Check sheet for the drawn part. Datum: minimum x, y, z corner. Units: mm. A direction names the side the tool comes from. Round coordinates to 2 decimals unless told otherwise and drop trailing zeros. Order: outer loops, then holes, each group sorted by start corner. A loop starts at its lowest first (then second) coordinate and runs counter-clockwise, first axis right, second up. Notation, with made-up numbers: (66.25, -32.5) - (119.25, -32.5) arc R5 cw to (119.25, -27.5) - close; hole circle Ø10 at (61, -33). An arc over 180 degrees is marked (long way). Write each question's results on one line, items separated by ' | '.
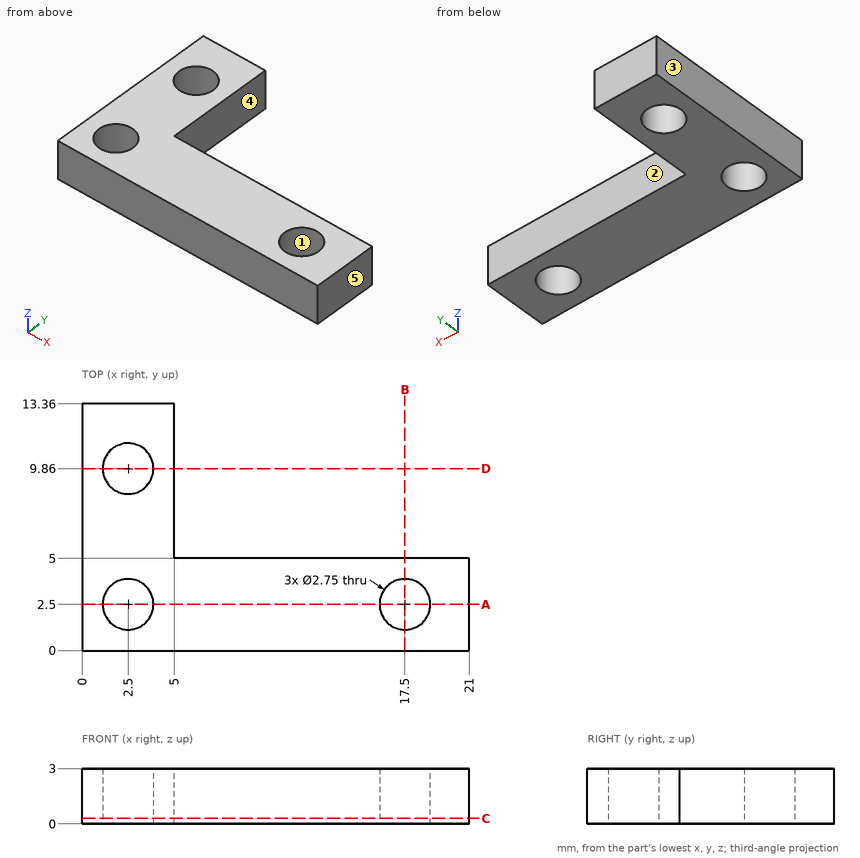
(1) Section check B-B (x = 17.5). Record the cut outline in (y, z) (3 decimals).
Answers follow:
outline: (0, 0) - (1.125, 0) - (1.125, 3) - (0, 3) - close; (3.875, 0) - (5, 0) - (5, 3) - (3.875, 3) - close
(2) Draft check along X on the marked faces 1, 2 and 3. Enter one of: released by +X, released by -X, zero draft, split by the parting line, or undercut.
Answers follow:
face 1: undercut | face 2: zero draft | face 3: released by -X
(3) Access from +Z, -Z, +X, -X, +Y, -Y to the whole of each face (thin tool, end or side, straight path). Record for the marked faces 4 and 5.
Answers follow:
face 4: +Z, -Z, +X, +Y | face 5: +Z, -Z, +X, +Y, -Y
(4) Section check A-A (y = 2.5). Record the cut outline in (x, z) (3 decimals), then the cut area to 3 significant figures.
Answers follow:
outline: (0, 0) - (1.125, 0) - (1.125, 3) - (0, 3) - close; (3.875, 0) - (16.125, 0) - (16.125, 3) - (3.875, 3) - close; (18.875, 0) - (21, 0) - (21, 3) - (18.875, 3) - close | area: 46.5 mm²
(5) Section check C-C (z = 0.3). Record the cut outline in (x, y) (3 decimals), then the cut area to 3 significant figures.
Answers follow:
outline: (0, 0) - (21, 0) - (21, 5) - (5, 5) - (5, 13.36) - (0, 13.36) - close; hole circle Ø2.75 at (2.5, 2.5); hole circle Ø2.75 at (2.5, 9.86); hole circle Ø2.75 at (17.5, 2.5) | area: 129 mm²
(6) Depth check by flat-ended pin: pin 1 Ø1.5 at (x, z) = (9, 1) entering from +Y. Enter the tip coordinate at first touch or a pass-through.
Answers follow:
pin 1: y = 5
(7) Material ranges on line 1 (Y direction, x = 2.5, z = 1.55) (3 decimals); line 2 (Y direction, x = 17.5, z = 1.3) (3 decimals); line 3 (X direction, y = 1.5, z = 2.7), recorded low to high.
Answers follow:
line 1: 0 to 1.125, 3.875 to 8.485, 11.235 to 13.36 | line 2: 0 to 1.125, 3.875 to 5 | line 3: 0 to 1.56, 3.44 to 16.56, 18.44 to 21
